Design review of the part built by this model. Coordinates are the model's own, in mm. Coordinates: 2 decimals unless noted, no trailing zeros. Loops run counter-clockwise (first coordinate to the right, second up) from the corner with the lowest first, then second, coordinate; pieces in that order, holes last. Notation, with made-up numbers: M -27,-38 L 22,-38 A18 cw 22,-25 Z; hole C -38,59.25 d1. An arc over 180 degrees is marked long. Write item = value, one per line. Start each with the question number.
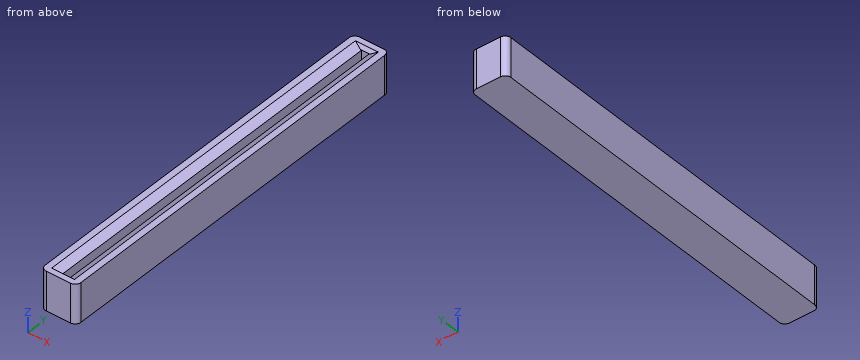
```python
from build123d import *

# Parameters (mm, degrees)
SKETCH2_W          = 10.033
SKETCH2_H          = 108.585
EXTRUDE2_DEPTH     = 10.9474
FILLET1_R          = 1.5875
SKETCH7_W          = 2.159
SKETCH7_H          = 104.14
CUT_EXTRUDE2_DEPTH = 6.731
CHAMFER1_SIZE      = 2.159
CHAMFER1_SIZE2     = 1.246499231
CHAMFER2_SIZE      = 0.635
CHAMFER2_SIZE2     = 1.099852263


with BuildPart() as part:
    # Sketch2 → Extrude2 (new body)
    with BuildSketch(Plane.XY):
        Rectangle(SKETCH2_W, SKETCH2_H)
    extrude(amount=EXTRUDE2_DEPTH)

    # Fillet1
    fillet1_edges = [part.edges().sort_by_distance(p)[0] for p in [
        (-5.0165, 54.2925, 5.4737),
        (5.0165, 54.2925, 5.4737),
        (5.0165, -54.2925, 5.4737),
        (-5.0165, -54.2925, 5.4737),
    ]]
    fillet(fillet1_edges, radius=FILLET1_R)

    # Sketch7 → Cut-Extrude2 (cut)
    with BuildSketch(Plane.XY.offset(10.9474)):
        Rectangle(SKETCH7_W, SKETCH7_H)
    extrude(amount=-CUT_EXTRUDE2_DEPTH, mode=Mode.SUBTRACT)

    # Chamfer1
    chamfer1_edges = [part.edges().sort_by_distance(p)[0] for p in [
        (-1.0795, 0, 10.9474),
        (1.0795, 0, 10.9474),
    ]]
    chamfer1_side = [part.faces().sort_by_distance(p)[0] for p in [
        (0, 53.202024722, 10.9474),
    ]]
    chamfer(chamfer1_edges, length=CHAMFER1_SIZE, length2=CHAMFER1_SIZE2, reference=chamfer1_side[0])

    # Chamfer2
    chamfer2_edges = [part.edges().sort_by_distance(p)[0] for p in [
        (0, 52.07, 10.9474),
        (0, -52.07, 10.9474),
    ]]
    chamfer2_side = [part.faces().sort_by_distance(p)[0] for p in [
        (0, 53.160475278, 10.9474),
    ]]
    chamfer(chamfer2_edges, length=CHAMFER2_SIZE, length2=CHAMFER2_SIZE2, reference=chamfer2_side[0])


solid = part.part
```
(1) Take a section at A-A (z = 6). State the section outline as (x, y) points (1 decimal).
(2) Take a section at B-B (y = 44.5). State the section outline as (x, z) points, plus the area to 3 significant figures.
(3) Insertion check: pin 1 (1.1 mm diameter, centred on x = 0, y = -6, fed in from +Z). The pin has a flat end and moves straight along its axis. Give the tip position at first contact, or say it passes through.
(4) To check wall thickness, follow L1, parallel to Y at x = 1, z = 9.25; L2, parallel to X at y = -37.5, z = 7.5; L3, parallel to Z at x = -0.25, y = -17. State the ranges of each line that lie inside material, in increasing order.
Results list:
q1.outline = M -5,-52.7 A1.6 ccw -3.4,-54.3 L 3.4,-54.3 A1.6 ccw 5,-52.7 L 5,52.7 A1.6 ccw 3.4,54.3 L -3.4,54.3 A1.6 ccw -5,52.7 Z; hole M -1.1,-52.1 L 1.1,-52.1 L 1.1,52.1 L -1.1,52.1 Z
q2.outline = M -5.02,0 L 5.02,0 L 5.02,10.95 L 3.24,10.95 L 1.08,9.7 L 1.08,4.22 L -1.08,4.22 L -1.08,9.7 L -3.24,10.95 L -5.02,10.95 Z
q2.area = 92.6 mm^2
q3.pin_1 = 4.22
q4.L1 = -54.29 to -52.07, 52.07 to 54.29
q4.L2 = -5.02 to -1.08, 1.08 to 5.02
q4.L3 = 0 to 4.22
